Source: CAD feature listing. Evaluate the final solid. Frame: model axes, mm. A direction names the side the tool comes from. Round coordinates to 2 decimals unless told otherwise and drop trailing zeros. Order: outer loops, then holes, each group sorted by start corner. A loop starts at its lowest first (then second) coordinate and runs counter-clockwise, first axis right, second up.
```python
from build123d import *

# Parameters (mm, degrees)
SKETCH1_R           = 52.3875
SKETCH1_W           = 120
SKETCH1_H           = 60
BOSS_EXTRUDE1_DEPTH = 190


with BuildPart() as part:
    # Sketch1 → Boss-Extrude1 (new body)
    with BuildSketch(Plane.XY):
        with BuildLine():
            Line((-70, -62.3875), (-70, -122.3875))
            ThreePointArc((-70, -122.3875), (-67.071067812, -129.458567812), (-60, -132.3875))
            Line((-60, -132.3875), (60, -132.3875))
            ThreePointArc((60, -132.3875), (67.071067812, -129.458567812), (70, -122.3875))
            Line((70, -122.3875), (70, -62.3875))
            ThreePointArc((70, -62.3875), (67.071067812, -55.316432188), (60, -52.3875))
            Line((60, -52.3875), (60, -17.093863117))
            ThreePointArc((60, -17.093863117), (0, 62.3875), (-60, -17.093863117))
            Line((-60, -17.093863117), (-60, -52.3875))
            ThreePointArc((-60, -52.3875), (-67.071067812, -55.316432188), (-70, -62.3875))
        make_face()
        Circle(SKETCH1_R, mode=Mode.SUBTRACT)
        with Locations((0, -92.3875)):
            Rectangle(SKETCH1_W, SKETCH1_H, mode=Mode.SUBTRACT)
    extrude(amount=BOSS_EXTRUDE1_DEPTH)


solid = part.part
```
1. Section C-C on y = 0. Return loops of the section in (x, z), plus the area to 3 significant figures.
2. Access query for faces 4 (the face through (70, -93, 94)), 5 (the face through (-70, -92, 94)), 6 (the face through (-60, -34, 94)), 7 (the face through (60, -35, 94)), 8 (the face through (60, -93, 94)). Directions: +Z, -Z, +X, -X, +Y, -Y. A direction counts if a zero-diameter tool reaches every point of the face in a straight line with its end or side. Return the directions, or none.
3. Section A-A on x = 0. Return loops of the section in (y, z), plus the area to 3 significant figures.
4. Section B-B on z = 95.5. Return loops of the section in (x, y) (1 decimal), plus the area to 3 significant figures.
5. Pull-direction query (X, two-part tool) for faces 1 (the face through (-1, -132.388, 94)), 2 (the face through (1.614, 62.367, 93.67)), 3 (the face through (-60, -93, 94)); classes: released by +X, released by -X, zero draft, split by the parting line, or undercut.
6. First-contact query: pin 1 (5 mm diameter, centred on y = 24.5, z = 93, fed in from -X); pin 2 (12 mm diameter, centred on x = -21, y = -70.5, fed in from +Z); pin 3 (6 mm diameter, centred on y = 24, z = 51.5, fed in from +X). Flat tips, straight axial feed; report the tip coordinate or a pass-through.
7. Section D-D on x = 22.5. Return loops of the section in (y, z), plus the area to 3 significant figures.
8. Line query: line 1 along Y through (x, z) = (0, 80); line 2 along Y through (x, z) = (-11, 95.5); line 3 along X through (y, z) = (-24, 9.5). Output: solid intervals per line, ascending.
Result:
1. outline: (-62.39, 0) - (-52.39, 0) - (-52.39, 190) - (-62.39, 190) - close; (52.39, 0) - (62.39, 0) - (62.39, 190) - (52.39, 190) - close
1. area: 3,800 mm2
2. face 4: +Z, -Z, +X, +Y, -Y
2. face 5: +Z, -Z, -X, +Y, -Y
2. face 6: +Z, -Z, -X
2. face 7: +Z, -Z, +X
2. face 8: +Z, -Z
3. outline: (-132.39, 0) - (-122.39, 0) - (-122.39, 190) - (-132.39, 190) - close; (-62.39, 0) - (-52.39, 0) - (-52.39, 190) - (-62.39, 190) - close; (52.39, 0) - (62.39, 0) - (62.39, 190) - (52.39, 190) - close
3. area: 5,700 mm2
4. outline: (-70, -122.4) arc R10 ccw to (-60, -132.4) - (60, -132.4) arc R10 ccw to (70, -122.4) - (70, -62.4) arc R10 ccw to (60, -52.4) - (60, -17.1) arc R62.4 ccw (long way) to (-60, -17.1) - (-60, -52.4) arc R10 ccw to (-70, -62.4) - close; hole (-60, -122.4) - (60, -122.4) - (60, -62.4) - (-60, -62.4) - close; hole circle Ø104.8 at (0, 0)
4. area: 7,750 mm2
5. face 1: zero draft
5. face 2: split by the parting line
5. face 3: undercut
6. pin 1: stops at x = -58.38
6. pin 2: passes through
6. pin 3: stops at x = 58.75
7. outline: (-132.39, 0) - (-122.39, 0) - (-122.39, 190) - (-132.39, 190) - close; (-62.39, 0) - (-47.31, 0) - (-47.31, 190) - (-62.39, 190) - close; (47.31, 0) - (58.19, 0) - (58.19, 190) - (47.31, 190) - close
7. area: 6,830 mm2
8. line 1: y = -132.39 to -122.39, -62.39 to -52.39, 52.39 to 62.39
8. line 2: y = -132.39 to -122.39, -62.39 to -51.22, 51.22 to 61.41
8. line 3: x = -60 to -46.57, 46.57 to 60
